from build123d import *

# Parameters (mm, degrees)
F1_DEPTH = 5
F3_DEPTH = 400
F5_D     = 5
F7_D     = 5
F8_W     = 5
F8_H     = 5
F9_DEPTH = 400


with BuildPart() as f1:
    # F0 (on Top) → F1 (new body)
    with BuildSketch(Plane.XY):
        Polygon((5, 0), (0, 0), (0, -10), (21, -10), (21, -5), (11, -5), (11, 0), (6, 0), align=None)
    extrude(amount=F1_DEPTH)

    # F2 (on face) → F3 (join)
    with BuildSketch(Plane.XY.offset(5)):
        Polygon((5, 0), (0, 0), (0, -10), (21, -10), (21, -5), (11, -5), (11, 0), (6, 0), (6, -5), (5, -5), align=None)
    extrude(amount=F3_DEPTH)

    # F5 (through all)
    with Locations(Plane(origin=(0, -5, 0), x_dir=(-1, 0, 0), z_dir=(0, 1, 0))):
        with Locations((-16, 10)):
            Hole(F5_D / 2)

    # F7 (through all)
    with Locations(Plane(origin=(0, -5, 0), x_dir=(-1, 0, 0), z_dir=(0, 1, 0))):
        with Locations((-16, 395)):
            Hole(F7_D / 2)

    # F8 (on face) → F9 (cut)
    with BuildSketch(Plane.XY.offset(405)):
        with Locations((8.5, -2.5)):
            Rectangle(F8_W, F8_H)
    extrude(amount=-F9_DEPTH, mode=Mode.SUBTRACT)


solid = f1.part
Can you work these out from the model? Positions are in its coordinate system, mm. Coordinates: 2 decimals unless noted, no trailing zeros. Write each loop counter-clockwise with the first axis right and the second up, starting at its lowest first coordinate (ties: lowest second). Pieces come first, ordered by that corner, then holes. Notation, with made-up numbers: (71, 59) -> (100, 59) arc R20 ccw to (100, 70) -> close; hole circle Ø6 at (81.25, -9.5). An arc over 180 degrees is marked (long way). Write each question's results on one line, items separated by ' | '. Start each with the question number.
Q1. I'm going to push flat-ended pins straight in: pin 1 (5.5 mm diameter, centred on x = 8, y = -2, fed in from +Z); pin 2 (2 mm diameter, centred on x = 8.5, z = 255.5, fed in from +Y); pin 3 (1.5 mm diameter, centred on y = -1.5, z = 259.5, fed in from +X). Where does each tip first touch, or does it pass through?
Q2. If I drill on probe 1 along Z at (x, y) = (16, -6.1); probe 2 along X at (y, z) = (-6.7, 395); probe 3 along Y at (x, z) = (15.75, 211), over which ranges is the centre line in solid material (lowest first)?
Q3. Imagine slicing it at A-A (z = 311). Write out the boundary of the cut face in (x, y).
Taken from the geometry:
1) pin 1: stops at z = 5 | pin 2: stops at y = -5 | pin 3: stops at x = 5
2) probe 1: z = 0 to 7.5, 12.5 to 392.5, 397.5 to 405 | probe 2: x = 0 to 13.5, 18.5 to 21 | probe 3: y = -10 to -5
3) outline: (0, -10) -> (21, -10) -> (21, -5) -> (5, -5) -> (5, 0) -> (0, 0) -> close
